Design review of the part built by this model. Coordinates are the model's own, in mm. A direction names the side the tool comes from. Give positions to 0.01 mm unless a question says otherwise; leave off trailing zeros. Write each loop counter-clockwise with the first axis right and the second up, starting at its lowest first coordinate (ties: lowest second). Pieces come first, ordered by that corner, then holes. Notation, with made-up numbers: (-5.5, 44) - (31.5, 44) arc R30 ccw to (31.5, 67) - close; hole circle Ø8 at (-32.5, 40.25). An arc over 180 degrees is marked (long way). Write each question's results on one line, items separated by ' | '. Start each with the question number.
from build123d import *

# Parameters (mm, degrees)
SKETCH1_W           = 31
SKETCH1_H           = 13
SKETCH1_R           = 1.25
BOSS_EXTRUDE1_DEPTH = 2
SKETCH2_W           = 31
SKETCH2_H           = 4.2
SKETCH2_W_2         = 27.6
SKETCH2_H_2         = 2.2
BOSS_EXTRUDE2_DEPTH = 4


with BuildPart() as part:
    # Sketch1 → Boss-Extrude1 (new body)
    with BuildSketch(Plane(origin=(0, 0, 0), x_dir=(1, 0, 0), z_dir=(0, 1, 0))):
        with Locations((15.5, 6.5)):
            Rectangle(SKETCH1_W, SKETCH1_H)
        with Locations(Location((4.5, 3.2, 0), (0, 0, 270))):
            Circle(SKETCH1_R, mode=Mode.SUBTRACT)
        with Locations(Location((26.5, 3.2, 0), (0, 0, 90))):
            Circle(SKETCH1_R, mode=Mode.SUBTRACT)
    extrude(amount=BOSS_EXTRUDE1_DEPTH)

    # Sketch2 → Boss-Extrude2 (add)
    with BuildSketch(Plane.XZ):
        with Locations((15.5, -7.8)):
            Rectangle(SKETCH2_W, SKETCH2_H)
        with Locations((15.5, -7.8)):
            Rectangle(SKETCH2_W_2, SKETCH2_H_2, mode=Mode.SUBTRACT)
    extrude(amount=BOSS_EXTRUDE2_DEPTH)


solid = part.part
Q1. Machinability: for faces 1 (the face through (15, 0, -8)), 2 (the face through (15, 0, -11)), 3 (the face through (15, 0, -3)), 4 (the face through (3.28, 0.99, -3.47)), which of the approach directions +Z, -Z, +X, -X, +Y, -Y give a long, thin tool a straight path to every point of the face, cutting with its end or side? Answer none if there is none.
Q2. Add section B-B on x = 26.5. State the section outline as (y, z) points, plus the area to 3 significant figures.
Q3. The part is to be moulded in two halves that separate along X. For faces 5 (the face through (1.7, -2, -8)), 6 (the face through (15, 2, -7)), 7 (the face through (31, 0, -6)), say which applies: +X half, -X half, draft (parallel to the pull), parting line (faces both ways), or undercut.
Q4. Insertion check: P1, Ø1.2, axis at x = 10.5, y = -1.5, coming from the +Z side; P2, Ø4, axis at x = 26.5, z = -3.2, coming from the -Y side; P3, Ø1.2, axis at x = 21, y = -2, coming from the -Z side. Each pin has a flat end and moves straight along its axis. Give the tip position at first contact, or say it passes through.
Q5. Add section C-C on z = -3.2. State the section outline as (x, y) points.
Q6. Add section D-D on x = 21. State the section outline as (y, z) points, plus the area to 3 significant figures.
Q7. Add section A-A on y = -1.3. State the section outline as (x, z) points.
Q8. For line 1 along X through (y, z) = (1, -3.2); line 2 along X through (y, z) = (-0.55, -7.25); line 3 along Z through (x, y) = (9, -0.4), list the stretches that pass through material, from the lowest coordinate up. Write a range as [from, to].
Result:
1) face 1: -Y | face 2: -Z, +X, -X, -Y | face 3: +Z, +X, -X, -Y | face 4: +Y, -Y
2) outline: (-4, -9.9) - (0, -9.9) - (0, -13) - (2, -13) - (2, -4.45) - (0, -4.45) - (0, -5.7) - (-4, -5.7) - (-4, -6.7) - (0, -6.7) - (0, -8.9) - (-4, -8.9) - close; (0, -1.95) - (2, -1.95) - (2, 0) - (0, 0) - close | area: 29.0 mm²
3) face 5: undercut | face 6: draft | face 7: +X half
4) P1: stops at z = -5.7 | P2: stops at y = 0 | P3: stops at z = -9.9
5) outline: (0, 0) - (3.25, 0) - (3.25, 2) - (0, 2) - close; (5.75, 0) - (25.25, 0) - (25.25, 2) - (5.75, 2) - close; (27.75, 0) - (31, 0) - (31, 2) - (27.75, 2) - close
6) outline: (-4, -9.9) - (0, -9.9) - (0, -13) - (2, -13) - (2, 0) - (0, 0) - (0, -5.7) - (-4, -5.7) - (-4, -6.7) - (0, -6.7) - (0, -8.9) - (-4, -8.9) - close | area: 34.0 mm²
7) outline: (0, -9.9) - (31, -9.9) - (31, -5.7) - (0, -5.7) - close; hole (1.7, -8.9) - (29.3, -8.9) - (29.3, -6.7) - (1.7, -6.7) - close
8) line 1: x = [0, 3.25], [5.75, 25.25], [27.75, 31] | line 2: x = [0, 1.7], [29.3, 31] | line 3: z = [-9.9, -8.9], [-6.7, -5.7]
